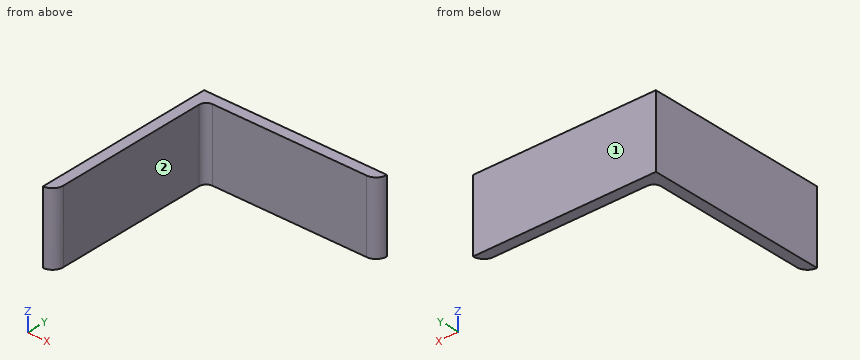
```python
from build123d import *

# Parameters (mm, degrees)
SALIENTE_EXTRUIR1_DEPTH = 20


with BuildPart() as part:
    # Croquis1 → Saliente-Extruir1 (new body)
    with BuildSketch(Plane.XY):
        with BuildLine():
            Line((22.208537854, 22.208537854), (-20.591462146, 22.208537854))
            ThreePointArc((-20.591462146, 22.208537854), (-22.005675708, 21.622751417), (-22.591462146, 20.208537854))
            Line((-22.591462146, 20.208537854), (-22.591462146, -22.591462146))
            ThreePointArc((-22.591462146, -22.591462146), (-23.470141802, -24.712782489), (-25.591462146, -25.591462146))
            Line((-25.591462146, -25.591462146), (-25.591462146, 25.208537854))
            Line((-25.591462146, 25.208537854), (25.208537854, 25.208537854))
            ThreePointArc((25.208537854, 25.208537854), (24.329858198, 23.087217511), (22.208537854, 22.208537854))
        make_face()
    extrude(amount=SALIENTE_EXTRUIR1_DEPTH)


solid = part.part
```
Geometry: final body of the model. Coordinates: model frame, mm. Face numbers are marked on the shaded views. A direction names the side the tool comes from. Round coordinates to 2 decimals unless told otherwise and drop trailing zeros. Order: outer loops, then holes, each group sorted by start corner. A loop starts at its lowest first (then second) coordinate and runs counter-clockwise, first axis right, second up. Notation, with made-up numbers: (87, -3.75) -> (146, -3.75) arc R15 ccw to (146, 5.25) -> close; hole circle Ø11 at (20, 83.5). An arc over 180 degrees is marked (long way). Use one line per item in the form item = value. Start each with the question number.
1. Cut plane C-C (y = -10). Return the cut outline in (x, z).
2. Pin query (flat end, axial travel): pin 1 Ø1 at (x, z) = (1, 4.5) entering from -Y. Return the tip coordinate at first contact, or that it passes through.
3. Reachability of the marked faces 1 and 2 from +Z, -Z, +X, -X, +Y, -Y: full face, straight path, thin tool, end or side. Return the list, or none.
4. Cut plane B-B (x = 1). Return the cut outline in (y, z).
5. Line query: probe 1 along Y at (x, z) = (-13, 16); probe 2 along X at (y, z) = (4.5, 8); probe 3 along Y at (x, z) = (-23, 10.5). Output: solid intervals per line, ascending.
6. Cut plane A-A (z = 6.5). Return the cut outline in (x, y).
Solution:
q1.outline = (-25.59, 0) -> (-22.59, 0) -> (-22.59, 20) -> (-25.59, 20) -> close
q2.pin_1 = 22.21
q3.face_1 = +Z, -Z, +X, -X, +Y
q3.face_2 = +Z, -Z, +X, -Y
q4.outline = (22.21, 0) -> (25.21, 0) -> (25.21, 20) -> (22.21, 20) -> close
q5.probe_1 = 22.21 to 25.21
q5.probe_2 = -25.59 to -22.59
q5.probe_3 = -24.1 to 25.21
q6.outline = (-25.59, -25.59) arc R3 ccw to (-22.59, -22.59) -> (-22.59, 20.21) arc R2 cw to (-20.59, 22.21) -> (22.21, 22.21) arc R3 ccw to (25.21, 25.21) -> (-25.59, 25.21) -> close
